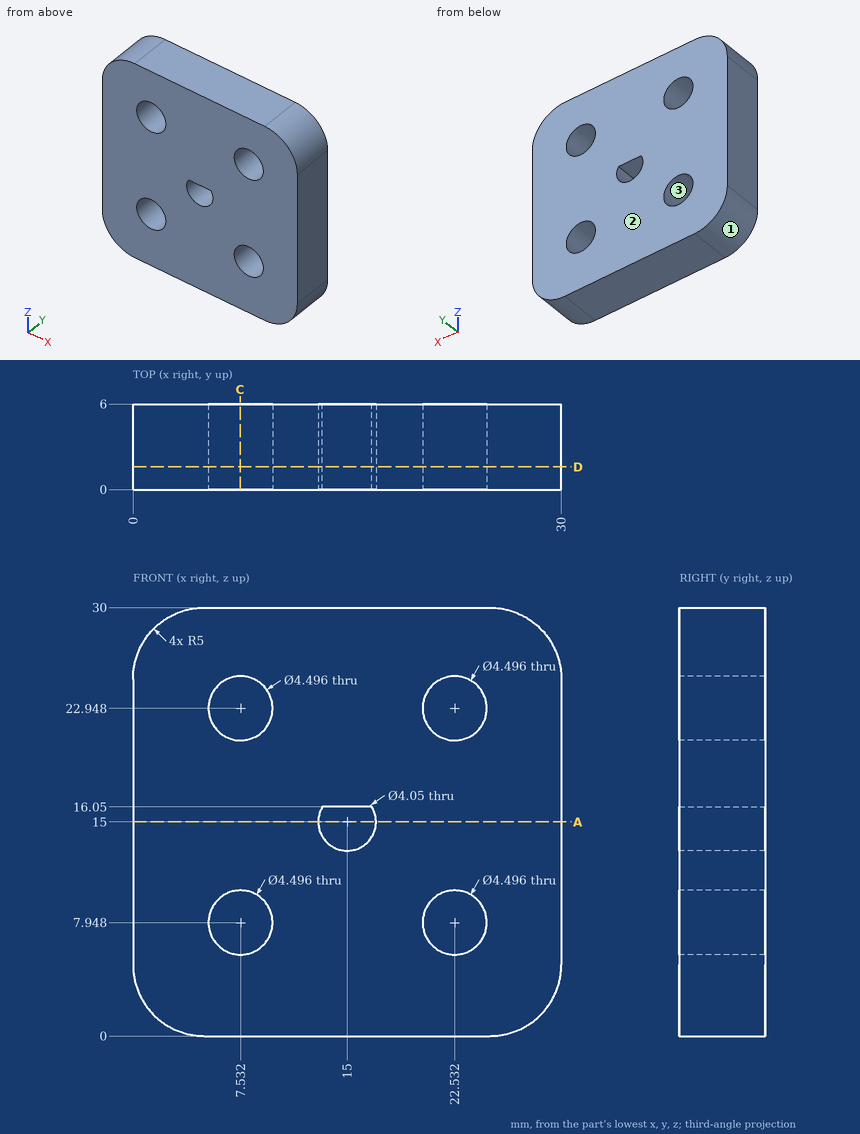
Job drawing, mm, ordinate dimensions from the low corner. One solid piece. Give positions to 0.01 mm unless a question says otherwise; leave off trailing zeros. Write each loop counter-clockwise with the first axis right and the second up, starting at its lowest first coordinate (ties: lowest second). Pieces come first, ordered by that corner, then holes. Notation, with made-up numbers: M 22,70.5 L 71,70.5 A28 ccw 71,95.5 Z; hole C -11,13.25 d6. An arc over 180 degrees is marked long. Put each result on its own line as item: value. Start each with the question number.
(1) Band-saw the part on D-D, the plane y = 1.6. Give the number of separate pieces and of enclosed holes in the cut face.
(2) Band-saw the part on A-A, the plane z = 15. Write the cut outline in (x, y) (1 decimal), and give its area (3 significant figures).
(3) Flat gauge pins, fed straight in: pin 1 Ø4 at (x, z) = (7.53, 22.95) entering from -Y; pin 2 Ø1.5 at (x, z) = (6, 27) entering from -Y. Where does each tip first touch, or does it go through?
(4) Probe L1, parallel to Z at x = 5.5, y = 1.35 (1 decimal); L2, parallel to X at y = 2, z = 24.75 (1 decimal); L3, parallel to X at y = 2.15, z = 21.25 (1 decimal). List the from-to ranges inside material, lowest first.
(5) Band-saw the part on C-C, the plane x = 7.5. Write the cut outline in (y, z).
(6) Mould opens along Z. For the marked faces 1, 2 and 3 say: +Z half, -Z half, draft (parallel to the pull), parting line (faces both ways), or undercut.
Response values:
1. separate pieces: 1
1. enclosed holes: 5
2. outline: M 0,0 L 13,0 L 13,6 L 0,6 Z; M 17,0 L 30,0 L 30,6 L 17,6 Z
2. area: 156 mm2
3. pin 1: passes through
3. pin 2: stops at y = 0
4. L1: z = 0 to 7, 8.9 to 22, 23.9 to 30
4. L2: x = 0 to 6.2, 8.9 to 21.2, 23.9 to 30
4. L3: x = 0 to 6.1, 9 to 21.1, 24 to 30
5. outline: M 0,0 L 6,0 L 6,5.7 L 0,5.7 Z; M 0,10.2 L 6,10.2 L 6,20.7 L 0,20.7 Z; M 0,25.2 L 6,25.2 L 6,30 L 0,30 Z
6. face 1: -Z half
6. face 2: draft
6. face 3: undercut
